Design review of the part shown in the three views and the two pictorial views. Dimensions are in mm from the part's minimum x, y and z. A direction names the side the tool comes from. Coordinates: 2 decimals unless noted, no trailing zeros. Write each loop counter-clockwise with the first axis right and the second up, starting at its lowest first coordinate (ties: lowest second). Pieces come first, ordered by that corner, then holes. Notation, with made-up numbers: (-21.5, -40) - (5.5, -40) arc R7 cw to (5.5, -31) - close; hole circle Ø7 at (43, 37). An arc over 180 degrees is marked (long way). Return JSON: item names as keys, results as strings. Group by question number.
(1) We need section D-D on x = 20.5. State the section outline as (y, z) points, then the cut area to 3 significant figures.
(2) We need section A-A on y = 45.1. State the section outline as (x, z) points, then the cut area to 3 significant figures.
(3) For pin 1 Ø1 at (x, z) = (7, 48.5) entering from -Y; pin 2 Ø7.5 at (x, y) = (12.7, 13.96) entering from +Z; pin 3 Ø4 at (x, z) = (8, 9.5) entering from +Y, all flat-tipped, find the tip position at first contact; note any pin that passes through.
(4) We need section C-C on y = 30.1. State the section outline as (x, z) points.
(5) We need section B-B on z = 46.5. Give the number of separate pieces and of enclosed holes in the cut face, then the cut area to 3 significant figures.
(6) Tool access review of the marked faces 1 and 2: name each direction out of +Z, -Z, +X, -X, +Y, -Y from which nothing blocks a thin tool from reaching the whole face with its end or side.
(7) To check wall thickness, follow L1, parallel to Y at x = 12.7, z = 52.6; L2, parallel to X at y = 45, z = 53; L3, parallel to Y at x = 13.25, z = 49. State the ranges of each line that lie inside material, in increasing order. Write a range as from..to.
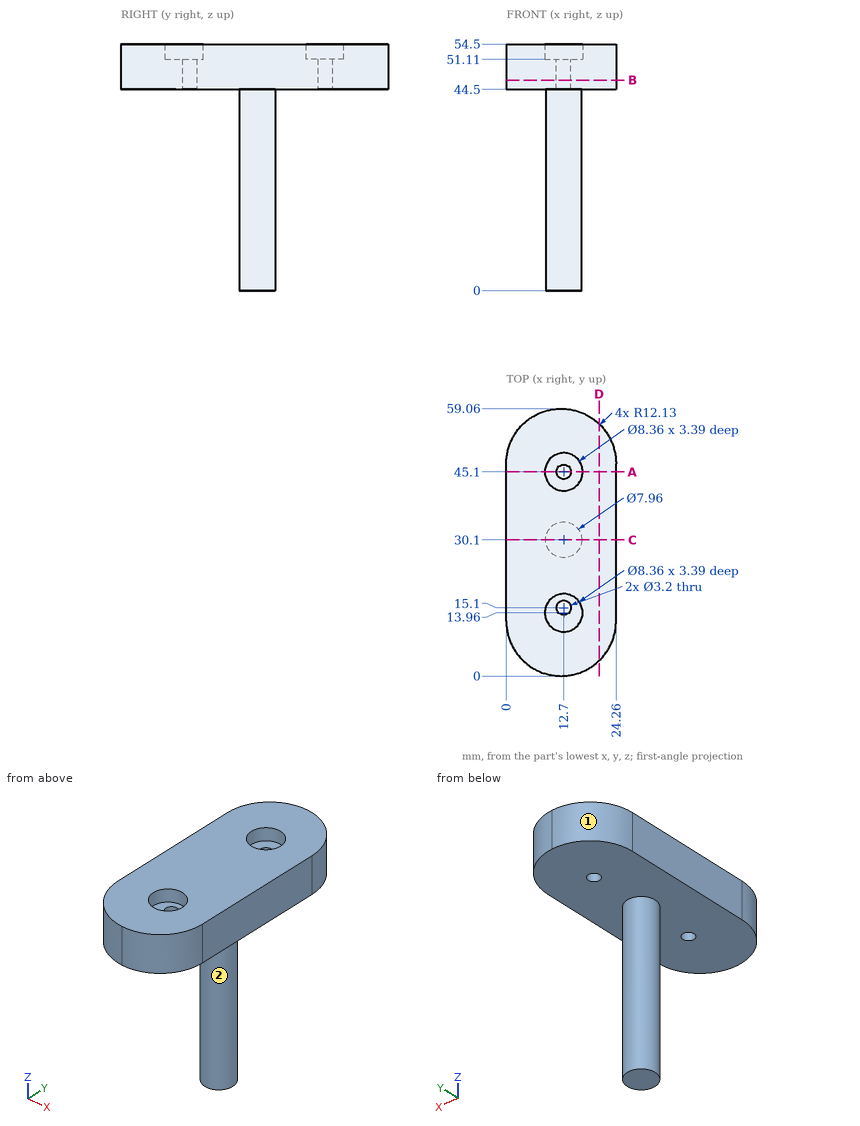
Ans:
{
 "1": {"outline": "(3.35, 44.5) - (55.71, 44.5) - (55.71, 54.5) - (3.35, 54.5) - close", "area": "524 mm²"},
 "2": {"outline": "(0, 44.5) - (11.1, 44.5) - (11.1, 51.11) - (8.52, 51.11) - (8.52, 54.5) - (0, 54.5) - close; (14.3, 44.5) - (24.26, 44.5) - (24.26, 54.5) - (16.88, 54.5) - (16.88, 51.11) - (14.3, 51.11) - close", "area": "193 mm²"},
 "3": {"pin 1": "y = 0.92", "pin 2": "z = 51.11", "pin 3": "y = 33.02"},
 "4": {"outline": "(0, 44.5) - (8.72, 44.5) - (8.72, 0) - (16.68, 0) - (16.68, 44.5) - (24.26, 44.5) - (24.26, 54.5) - (0, 54.5) - close"},
 "5": {"separate pieces": "1", "enclosed holes": "2", "area": "1,290 mm²"},
 "6": {"face 1": "+Z, -Z, -X, +Y", "face 2": "-Z"},
 "7": {"L1": "0.01..9.78, 18.14..40.92, 49.28..59.05", "L2": "0..8.52, 16.88..24.26", "L3": "0.05..13.6, 16.6..43.6, 46.6..59.01"}
}
